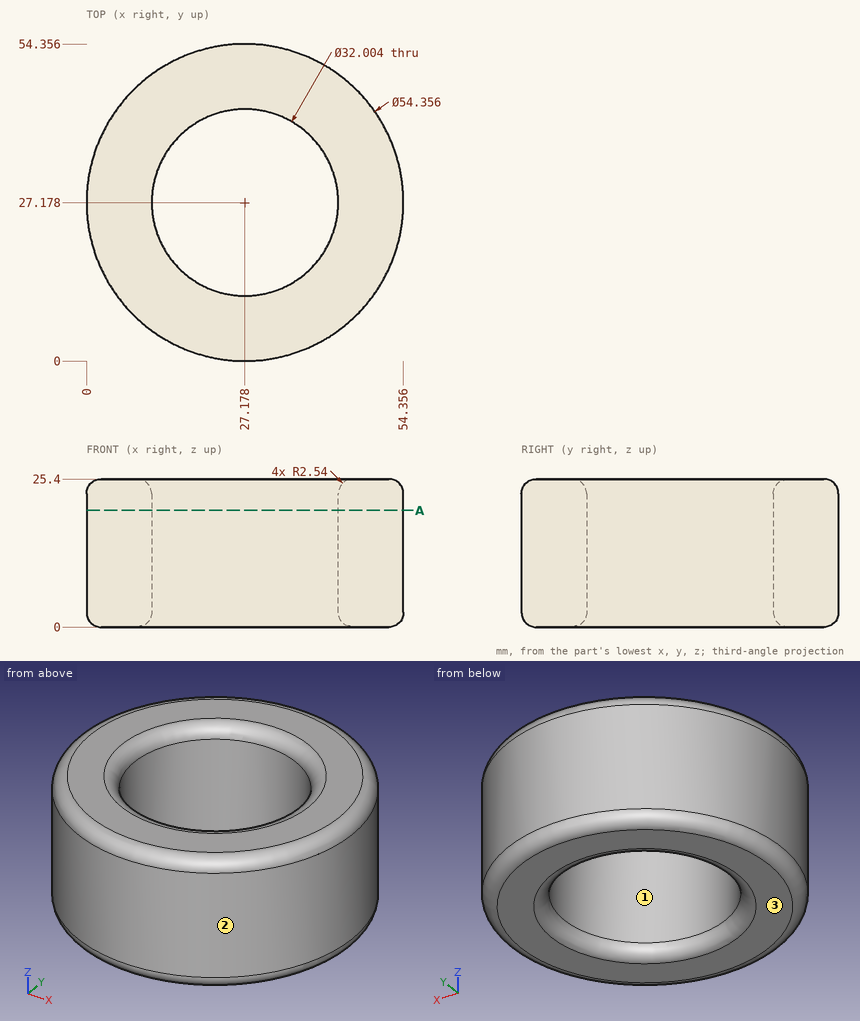
Could you check a few things on this drawing? It's one solid part, dimensions in mm from its lowest x, y, z. Give positions to 0.01 mm unless a question says otherwise; leave off trailing zeros. Order: outer loops, then holes, each group sorted by start corner. A loop starts at its lowest first (then second) coordinate and runs counter-clockwise, first axis right, second up.
1. Thinking about a two-plate mould opening in Y: for the marked faces 1, 2 and 3, which applies, +Y half, -Y half, draft (parallel to the pull), parting line (faces both ways), or undercut?
Answers below:
face 1: undercut
face 2: parting line
face 3: draft
2. Suppose I cut it at A-A (z = 20). Write out the boundary of the cut face in (x, y).
Answers below:
outline: circle Ø54.36 at (27.18, 27.18); hole circle Ø32 at (27.18, 27.18)
3. I need wall thicknesses on L1, parallel to Y at x = 25, z = 9.75; L2, parallel to X at y = 24, z = 5.5; L3, parallel to Y at x = 21, z = 21. Which ranges of each line are inside material? Lowest first, please.
Answers below:
L1: y = 0.09 to 11.32, 43.03 to 54.27
L2: x = 0.19 to 11.49, 42.86 to 54.17
L3: y = 0.71 to 12.42, 41.94 to 53.64
4. For pin 1 (1.5 mm diameter, centred on y = 6.5, z = 16, fed in from -X); pin 2 (4 mm diameter, centred on x = 16.5, z = 7, fed in from +Y); pin 3 (1.5 mm diameter, centred on y = 38.5, z = 15.5, fed in from +X), each with a flat end and sliding along its axis, tell me the tip position at first contact or that it passes through.
Answers below:
pin 1: stops at x = 8.7
pin 2: stops at y = 52.93
pin 3: stops at x = 52.22
